Input: part model. Units: mm. Frame: model coordinates. A direction names the side the tool comes from. Give positions to 0.01 mm unless a question says otherwise; leave off trailing zeros. Loops run counter-clockwise (first coordinate to the right, second up) from the corner with the lowest first, then second, coordinate; pieces in that order, holes last. Notation, with made-up numbers: (14, -30.5) -> (73, -30.5) arc R15 cw to (73, -10.5) -> close; hole circle Ø8 at (54.5, 75.5). An arc over 180 degrees is marked (long way). Answer as a JSON object with one key per item and string values.
Autodesk Inventor part; units mm, degrees
ref_plane "YZ Plane" through (0, 0, 0) normal (1, 0, 0) x (0, 1, 0)
ref_plane "XZ Plane" through (0, 0, 0) normal (0, 1, 0) x (-1, 0, 0)
ref_plane "XY Plane" through (0, 0, 0) normal (0, 0, 1) x (1, 0, 0)
sketch "Boceto1" plane through (0, 0, 0) normal (0, 0, 1) x (1, 0, 0)
  line L0 (-2.75, 1.5839) -> (-0.0033, 3.1735)
  line L1 (-0.0033, 3.1735) -> (2.7467, 1.5896)
  line L2 (2.7467, 1.5896) -> (2.75, -1.5839)
  line L3 (2.75, -1.5839) -> (0.0033, -3.1735)
  line L4 (0.0033, -3.1735) -> (-2.7467, -1.5896)
  line L5 (-2.7467, -1.5896) -> (-2.75, 1.5839)
  point P0 (0, 0)
  point P1 (0, 0)
extrude "Extrusión1" add sketch "Boceto1" against normal blind 2
sketch "Boceto2" plane through (0, 0, -2) normal (0, 0, -1) x (-1, 0, 0)
  circle A0 centre (0, 0) radius 1.5
  dimension "d3" = 3
extrude "Extrusión2" add sketch "Boceto2" along normal blind 12
properties part number "Tornillo para Bracket"
Q1. Access query for faces 1 (the flat face through (-1.396, 2.368, -0.986)), 2 (the flat face through (-1.3, -1.4, -2)). Directions: +Z, -Z, +X, -X, +Y, -Y. A direction counts if a zero-diameter tool reaches every point of the face in a straight line with its end or side. Return the directions, or none.
Evaluation:
{"face 1": "+Z, -Z, -X, +Y", "face 2": "-Z"}
Q2. Ray query, line 1 along Z through (x, y) = (-0.3, 2); line 2 along Y through (x, z) = (-1.1, -4); line 3 along Y through (x, z) = (-0.7, -10). Return the intervals inside material, ascending.
Evaluation:
{"line 1": "z = -2 to 0", "line 2": "y = -1.02 to 1.02", "line 3": "y = -1.33 to 1.33"}
Q3. Section D-D, the plane y = -2. Return the cut outline in (x, z).
Evaluation:
{"outline": "(-2.03, -2) -> (2.03, -2) -> (2.03, 0) -> (-2.03, 0) -> close"}
Q4. Pin query (flat end, axial travel): pin 1 (1.5 mm diameter, centred on x = -1.5, z = -7.5, fed in from -Y); pin 2 (1 mm diameter, centred on y = -1.5, z = -4.5, fed in from -X); pin 3 (1 mm diameter, centred on y = -0.5, z = -6, fed in from +X). Return the tip coordinate at first contact, or that it passes through.
Evaluation:
{"pin 1": "stops at y = -1.3", "pin 2": "stops at x = -1.12", "pin 3": "stops at x = 1.5"}
Q5. Section B-B, the plane x = 0.7. Return the cut outline in (y, z), then the cut area to 3 significant figures.
Evaluation:
{"outline": "(-2.77, -2) -> (-1.33, -2) -> (-1.33, -14) -> (1.33, -14) -> (1.33, -2) -> (2.77, -2) -> (2.77, 0) -> (-2.77, 0) -> close", "area": "42.9 mm2"}
Q6. Section A-A, the plane y = 1.25. Return the cut outline in (x, z), then the cut area to 3 significant figures.
Evaluation:
{"outline": "(-2.75, -2) -> (-0.83, -2) -> (-0.83, -14) -> (0.83, -14) -> (0.83, -2) -> (2.75, -2) -> (2.75, 0) -> (-2.75, 0) -> close", "area": "30.9 mm2"}
Q7. Section C-C, the plane z = -11.75. Return the cut outline in (x, y), then the cut area to 3 significant figures.
Evaluation:
{"outline": "circle Ø3 at (0, 0)", "area": "7.07 mm2"}
